The listing builds one solid part. Answer for the finished solid, in the listing's coordinates (mm). A direction names the side the tool comes from. Coordinates: 2 decimals unless noted, no trailing zeros. Order: outer loops, then holes, each group sorted by start corner. A loop starts at its lowest first (then second) coordinate and runs counter-clockwise, first axis right, second up. Notation, with made-up numbers: (88.25, 45) -> (124.25, 45) arc R14 ccw to (124.25, 58) -> close; hole circle Ø3 at (19.5, 12.25). An arc over 180 degrees is marked (long way). Write item = value, one per line.
from build123d import *

# Parameters (mm, degrees)
BASE_FLANGE2_DEPTH = 118.872
SKETCH3_R          = 2.54
CUT_EXTRUDE1_DEPTH = 2.286
SKETCH4_R          = 2.3876
CUT_EXTRUDE3_DEPTH = 2.286
SKETCH7_R          = 2.38125
CUT_EXTRUDE4_DEPTH = 2.286


# Sheet-metal steps are written as plain solids
with BuildPart() as part:
    # Sketch2 → Base-Flange2 (new body)
    with BuildSketch(Plane.XY):
        with BuildLine():
            Line((16.51, 404.114), (2.4384, 404.114))
            ThreePointArc((2.4384, 404.114), (0.714190825, 403.399809175), (0, 401.6756))
            Line((0, 401.6756), (0, 2.4384))
            ThreePointArc((0, 2.4384), (0.714190825, 0.714190825), (2.4384, 0))
            Line((2.4384, 0), (16.51, 0))
            Line((16.51, 0), (16.51, 2.286))
            Line((16.51, 2.286), (2.4384, 2.286))
            ThreePointArc((2.4384, 2.286), (2.330636927, 2.330636927), (2.286, 2.4384))
            Line((2.286, 2.4384), (2.286, 401.6756))
            ThreePointArc((2.286, 401.6756), (2.330636927, 401.783363073), (2.4384, 401.828))
            Line((2.4384, 401.828), (16.51, 401.828))
            Line((16.51, 401.828), (16.51, 404.114))
        make_face()
    extrude(amount=BASE_FLANGE2_DEPTH)

    # Sketch3 → Cut-Extrude1 (cut)
    with BuildSketch(Plane.ZY):
        with Locations((5.715, 258.064)):
            Circle(SKETCH3_R)
        with Locations((113.157, 258.064)):
            Circle(SKETCH3_R)
        with Locations((5.715, 143.764)):
            Circle(SKETCH3_R)
        with Locations((113.157, 143.764)):
            Circle(SKETCH3_R)
        with Locations((5.715, 372.364)):
            Circle(SKETCH3_R)
        with Locations((113.157, 372.364)):
            Circle(SKETCH3_R)
        with Locations((113.157, 29.464)):
            Circle(SKETCH3_R)
        with Locations((5.715, 29.464)):
            Circle(SKETCH3_R)
    extrude(amount=-CUT_EXTRUDE1_DEPTH, mode=Mode.SUBTRACT)

    # Sketch4 → Cut-Extrude3 (cut)
    with BuildSketch(Plane.XZ):
        with Locations(Location((9.906, 107.061, 0), (0, 0, 270))):
            Circle(SKETCH4_R)
        with Locations(Location((9.906, 11.811, 0), (0, 0, 270))):
            Circle(SKETCH4_R)
    extrude(amount=-CUT_EXTRUDE3_DEPTH, mode=Mode.SUBTRACT)

    # Sketch7 → Cut-Extrude4 (cut)
    with BuildSketch(Plane(origin=(0, 404.114, 0), x_dir=(-1, 0, 0), z_dir=(0, 1, 0))):
        with Locations(Location((-9.906, 103.886, 0), (0, 0, 90))):
            Circle(SKETCH7_R)
        with Locations(Location((-9.906, 14.986, 0), (0, 0, 90))):
            Circle(SKETCH7_R)
    extrude(amount=-CUT_EXTRUDE4_DEPTH, mode=Mode.SUBTRACT)


solid = part.part
Q1. Find the intervals of material crossed by line 1 along Y through (x, z) = (13.5, 104.5); line 2 along X through (y, z) = (82.5, 69.5), in increasing order.
The answers:
line_1 = 0 to 2.29, 401.83 to 404.11
line_2 = 0 to 2.29
Q2. The mould has two halves that part along Y. Classify faces 3 (the face through (10, 2.286, 59)), 4 (the face through (1, 203, 0)), 5 (the face through (10, 404.114, 59)), 6 (the face through (9, 0, 59)): released by +Y, released by -Y, zero draft, split by the parting line, or undercut.
The answers:
face_3 = undercut
face_4 = zero draft
face_5 = released by +Y
face_6 = released by -Y
Q3. Section A-A, the plane z = 41 is taken. Give the vertices of the cut face in (x, y), plus the area to 3 significant figures.
The answers:
outline = (0, 2.44) arc R2.44 ccw to (2.44, 0) -> (16.51, 0) -> (16.51, 2.29) -> (2.44, 2.29) arc R0.15 cw to (2.29, 2.44) -> (2.29, 401.68) arc R0.15 cw to (2.44, 401.83) -> (16.51, 401.83) -> (16.51, 404.11) -> (2.44, 404.11) arc R2.44 ccw to (0, 401.68) -> close
area = 986 mm2
Q4. A tool of negligible diameter and unlimited length cuts with its end or side. For faces 1 (the face through (2.286, 199, 59)), 2 (the face through (0, 205, 59)), from which of +Z, -Z, +X, -X, +Y, -Y can it reach the whole face along a straight path? Write none if from no direction.
The answers:
face_1 = +Z, -Z, +X
face_2 = +Z, -Z, -X, +Y, -Y
Q5. Section B-B, the plane y = 356 is taken. Give the vertices of the cut face in (x, z), plus the area to 3 significant figures.
The answers:
outline = (0, 0) -> (2.29, 0) -> (2.29, 118.87) -> (0, 118.87) -> close
area = 272 mm2
Q6. Each of these flat-tipped pins is pushed along its axis until it touches: pin 1 Ø6 at (y, z) = (258.064, 113.157) entering from -X; pin 2 Ø1 at (y, z) = (118, 69) entering from +X; pin 3 Ø4.5 at (x, z) = (9.906, 11.811) entering from -Y. Where does it stop, or does it pass through?
The answers:
pin_1 = 0
pin_2 = 2.29
pin_3 = 401.83
